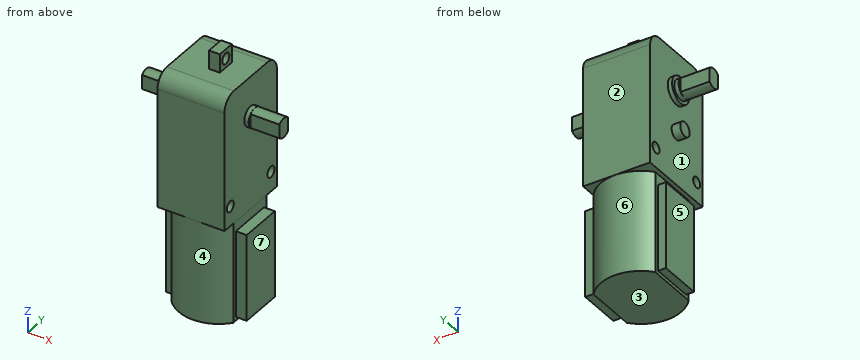
```python
from build123d import *

# Parameters (mm, degrees)
SKETCH1_W            = 37
SKETCH1_H            = 22.4
BOSS_EXTRUDE1_DEPTH  = 18.6
FILLET1_R            = 4
SKETCH2_R            = 3.65
BOSS_EXTRUDE2_DEPTH  = 1.2
SKETCH3_R            = 2.73
BOSS_EXTRUDE3_DEPTH  = 1.2
BOSS_EXTRUDE4_DEPTH  = 8
SKETCH5_R            = 2.72
BOSS_EXTRUDE5_DEPTH  = 1.2
BOSS_EXTRUDE6_DEPTH  = 8
SKETCH7_R            = 2
BOSS_EXTRUDE7_DEPTH  = 2.4
SKETCH8_W            = 5.14
SKETCH8_H            = 5.12
BOSS_EXTRUDE8_DEPTH  = 1.5
BOSS_EXTRUDE10_DEPTH = 28
SKETCH12_W           = 24
SKETCH12_H           = 12
BOSS_EXTRUDE11_DEPTH = 3
SKETCH13_R           = 1.5
CUT_EXTRUDE1_DEPTH   = 28
SKETCH14_R           = 1.5
CUT_EXTRUDE2_DEPTH   = 28


with BuildPart() as part:
    # Sketch1 → Boss-Extrude1 (new body)
    with BuildSketch(Plane(origin=(0, 0, 0), x_dir=(0, 0, -1), z_dir=(1, 0, 0))):
        Rectangle(SKETCH1_W, SKETCH1_H)
    extrude(amount=BOSS_EXTRUDE1_DEPTH)

    # Fillet1
    fillet1_edges = [part.edges().sort_by_distance(p)[0] for p in [
        (9.3, 11.2, 18.5),
        (9.3, -11.2, 18.5),
    ]]
    fillet(fillet1_edges, radius=FILLET1_R)

    # Sketch2 → Boss-Extrude2 (add)
    with BuildSketch(Plane.ZY):
        with Locations(Location((7.5, 0, 0), (0, 0, 180))):
            Circle(SKETCH2_R)
    extrude(amount=BOSS_EXTRUDE2_DEPTH)

    # Sketch3 → Boss-Extrude3 (add)
    with BuildSketch(Plane.ZY.offset(1.2)):
        with Locations((7.5, 0)):
            Circle(SKETCH3_R)
    extrude(amount=BOSS_EXTRUDE3_DEPTH)

    # Sketch4 → Boss-Extrude4 (add)
    with BuildSketch(Plane.ZY.offset(2.4)):
        with BuildLine():
            Line((5.552798511, -1.85), (9.447201489, -1.85))
            ThreePointArc((9.447201489, -1.85), (10.185906483, 0), (9.447201489, 1.85))
            Line((9.447201489, 1.85), (5.552798511, 1.85))
            ThreePointArc((5.552798511, 1.85), (4.814093517, 0), (5.552798511, -1.85))
        make_face()
    extrude(amount=BOSS_EXTRUDE4_DEPTH)

    # Sketch5 → Boss-Extrude5 (add)
    with BuildSketch(Plane(origin=(18.6, 0, 0), x_dir=(0, 0, -1), z_dir=(1, 0, 0))):
        with Locations((-7.5, 0)):
            Circle(SKETCH5_R)
    extrude(amount=BOSS_EXTRUDE5_DEPTH)

    # Sketch6 → Boss-Extrude6 (add)
    with BuildSketch(Plane(origin=(19.8, 0, 0), x_dir=(0, 0, -1), z_dir=(1, 0, 0))):
        with BuildLine():
            Line((-9.419930554, -1.85), (-5.580069446, -1.85))
            ThreePointArc((-5.580069446, -1.85), (-4.833797957, 0), (-5.580069446, 1.85))
            Line((-5.580069446, 1.85), (-9.419930554, 1.85))
            ThreePointArc((-9.419930554, 1.85), (-10.166202043, 0), (-9.419930554, -1.85))
        make_face()
    extrude(amount=BOSS_EXTRUDE6_DEPTH)

    # Sketch7 → Boss-Extrude7 (add)
    with BuildSketch(Plane.ZY):
        with Locations(Location((-3.9, 0, 0), (0, 0, 180))):
            Circle(SKETCH7_R)
    extrude(amount=BOSS_EXTRUDE7_DEPTH)

    # Sketch8 → Boss-Extrude8 (add, symmetric)
    with BuildSketch(Plane.ZY.offset(-10.2)):
        with Locations((21.07, 0)):
            Rectangle(SKETCH8_W, SKETCH8_H)
    extrude(amount=BOSS_EXTRUDE8_DEPTH, both=True)

    # Sketch11 → Boss-Extrude10 (add)
    with BuildSketch(Plane(origin=(0, 0, -18.5), x_dir=(-1, 0, 0), z_dir=(0, 0, -1))):
        with BuildLine():
            Line((-18.4, 7.128036195), (-18.4, -7.128036195))
            ThreePointArc((-18.4, -7.128036195), (-9.8, -11.17), (-1.2, -7.128036195))
            Line((-1.2, -7.128036195), (-1.2, 7.128036195))
            ThreePointArc((-1.2, 7.128036195), (-9.8, 11.17), (-18.4, 7.128036195))
        make_face()
    extrude(amount=BOSS_EXTRUDE10_DEPTH)

    # Sketch12 → Boss-Extrude11 (add)
    with BuildSketch(Plane(origin=(18.4, 0, 0), x_dir=(0, 0, -1), z_dir=(1, 0, 0))):
        with Locations((33.5, 0)):
            Rectangle(SKETCH12_W, SKETCH12_H)
    boss_extrude11 = extrude(amount=BOSS_EXTRUDE11_DEPTH)

    # Mirror1: Boss-Extrude11 across plane
    add(boss_extrude11.mirror(Plane.ZY.offset(-10.2)))

    # Sketch13 → Cut-Extrude1 (cut)
    with BuildSketch(Plane(origin=(18.6, 0, 0), x_dir=(0, 0, -1), z_dir=(1, 0, 0))):
        with Locations((13, -8.7)):
            Circle(SKETCH13_R)
    cut_extrude1 = extrude(amount=-CUT_EXTRUDE1_DEPTH, mode=Mode.SUBTRACT)

    # Mirror2: Cut-Extrude1 across plane
    add(cut_extrude1.mirror(Plane.ZX), mode=Mode.SUBTRACT)

    # Sketch14 → Cut-Extrude2 (cut)
    with BuildSketch(Plane.ZY.offset(-8.7)):
        with Locations((21.04, 0)):
            Circle(SKETCH14_R)
    extrude(amount=-CUT_EXTRUDE2_DEPTH, mode=Mode.SUBTRACT)


solid = part.part
```
For this review, take the finished solid that the model builds, in its own axes (mm). Face numbers are marked on the shaded views. A direction names the side the tool comes from. Round coordinates to 2 decimals unless told otherwise and drop trailing zeros. Write each loop counter-clockwise with the first axis right and the second up, starting at its lowest first coordinate (ties: lowest second). Pieces come first, ordered by that corner, then holes. Notation, with made-up numbers: (54.25, 24) - (106.25, 24) arc R23 ccw to (106.25, 36) - close; hole circle Ø2 at (84, -23.5). An arc over 180 degrees is marked (long way). Write each question's results on one line, items separated by ' | '.
Item 1: To check wall thickness, follow line 1 along Y through (x, z) = (4, -13); line 2 along Y through (x, z) = (10, 21); line 3 along X through (y, z) = (4.25, -17). State the ranges of each line that lie inside material, in increasing order. Write a range as from..to.
Calculated:
line 1: y = -11.2..-10.2, -7.2..7.2, 10.2..11.2 | line 2: y = -2.56..-1.5, 1.5..2.56 | line 3: x = 0..18.6
Item 2: Take a section at C-C on x = 10. Count the separate pieces of the cut face and the enclosed holes in it, then the cut area to 3 significant figures.
Calculated:
separate pieces: 1 | enclosed holes: 3 | area: 1,450 mm^2
Item 3: For pin 1 (1.5 mm diameter, centred on y = -5, z = -18.5, fed in from +X); pin 2 (1.8 mm diameter, centred on x = 0.5, z = -28.5, fed in from +Y); pin 3 (2 mm diameter, centred on y = 1, z = -3.5, fed in from -X); pin 4 (4 mm diameter, centred on x = 1, y = -7, fed in from -Z), all flat-tipped, find the tip position at first contact; note any pin that passes through.
Calculated:
pin 1: stops at x = 18.6 | pin 2: stops at y = 7.36 | pin 3: stops at x = -2.4 | pin 4: stops at z = -46.5
Item 4: Draft analysis for pull direction Z (two halves, no side actions). For the marked faces 1, 2 and 3, state which applies: pulls with the +Z half, pulls with the -Z half, needs draft (parallel to the pull), parting line crosses it, or undercut.
Calculated:
face 1: undercut | face 2: needs draft | face 3: pulls with the -Z half
Item 5: Take a section at A-A on z = 21.04. State the section outline as (x, y) points, then the cut area to 3 significant figures.
Calculated:
outline: (8.7, -2.56) - (11.7, -2.56) - (11.7, -1.5) - (8.7, -1.5) - close; (8.7, 1.5) - (11.7, 1.5) - (11.7, 2.56) - (8.7, 2.56) - close | area: 6.36 mm^2
Item 6: For the marked faces 4, 5, 6 and 7, list the 3-axis set-ups (+Z, -Z, +X, -X, +Y, -Y) from which the entire face can be reached by the end or side of a thin tool; tool diameter is ignored.
Calculated:
face 4: -Z, -Y | face 5: -Z, -X, +Y, -Y | face 6: -Z, +Y | face 7: -Z, +X, +Y, -Y
Item 7: Take a section at B-B on z = -13. State the section outline as (x, y) points, then the cut area to 3 significant figures.
Calculated:
outline: (0, -11.2) - (18.6, -11.2) - (18.6, -10.2) - (0, -10.2) - close; (0, -7.2) - (18.6, -7.2) - (18.6, 7.2) - (0, 7.2) - close; (0, 10.2) - (18.6, 10.2) - (18.6, 11.2) - (0, 11.2) - close | area: 305 mm^2
Item 8: Take a section at D-D on y = -8.7. State the section outline as (x, z) points, then the cut area to 3 significant figures.
Calculated:
outline: (0, -18.5) - (2.79, -18.5) - (2.79, -46.5) - (16.81, -46.5) - (16.81, -18.5) - (18.6, -18.5) - (18.6, -14.5) - (0, -14.5) - close; (0, -11.5) - (18.6, -11.5) - (18.6, 18.21) - (0, 18.21) - close | area: 1,020 mm^2
